Design review of the part built by this model. Coordinates are the model's own, in mm. Face numbers are marked on the shaded views. Coordinates: 2 decimals unless noted, no trailing zeros. Order: outer loops, then holes, each group sorted by start corner. A loop starts at its lowest first (then second) coordinate and runs counter-clockwise, first axis right, second up. Notation, with made-up numbers: (16, 12) -> (52, 12) arc R12 ccw to (52, 18) -> close; hole circle Ø5 at (86.25, 1.25). An arc over 180 degrees is marked (long way). Write item = value, one per line.
```python
from build123d import *

# Parameters (mm, degrees)
SKETCH_1_W          = 48.12
SKETCH_1_H          = 12
SKETCH_1_R          = 0.85
SKETCH_1_W_2        = 5
EXTRUDE_1_DEPTH     = 1.6
CUT_EXTRUDE_1_DEPTH = 1.6
FILLET_1_R          = 1


with BuildPart() as part:
    # 草图1 → 凸台-拉伸1 (new body)
    # profile 1 of 2: a face of its own
    with BuildSketch(Plane.XY):
        with Locations((29.06, -6)):
            Rectangle(SKETCH_1_W, SKETCH_1_H)
        with Locations((50.62, -9)):
            Circle(SKETCH_1_R, mode=Mode.SUBTRACT)
        with Locations((50.62, -3)):
            Circle(SKETCH_1_R, mode=Mode.SUBTRACT)
    # profile 2 of 2: a face of its own
    with BuildSketch(Plane.XY):
        with Locations((2.5, -6)):
            Rectangle(SKETCH_1_W_2, SKETCH_1_H)
        with Locations((2.5, -9)):
            Circle(SKETCH_1_R, mode=Mode.SUBTRACT)
        with Locations((2.5, -3)):
            Circle(SKETCH_1_R, mode=Mode.SUBTRACT)
    extrude(amount=EXTRUDE_1_DEPTH)

    # 草图2 → 切除-拉伸1 (cut)
    with BuildSketch(Plane(origin=(0, 0, 0), x_dir=(-1, 0, 0), z_dir=(0, 0, -1))):
        with BuildLine():
            Line((-42.930819808, -3), (-10.189180192, -3))
            ThreePointArc((-10.189180192, -3), (-7.189180192, -6), (-10.189180192, -9))
            Line((-10.189180192, -9), (-42.930819808, -9))
            ThreePointArc((-42.930819808, -9), (-45.930819808, -6), (-42.930819808, -3))
        make_face()
    extrude(amount=-CUT_EXTRUDE_1_DEPTH, mode=Mode.SUBTRACT)

    # 圆角1
    fillet_1_edges = [part.edges().sort_by_distance(p)[0] for p in [
        (53.12, -12, 0.8),
        (0, -12, 0.8),
        (0, 0, 0.8),
        (53.12, 0, 0.8),
    ]]
    fillet(fillet_1_edges, radius=FILLET_1_R)


solid = part.part
```
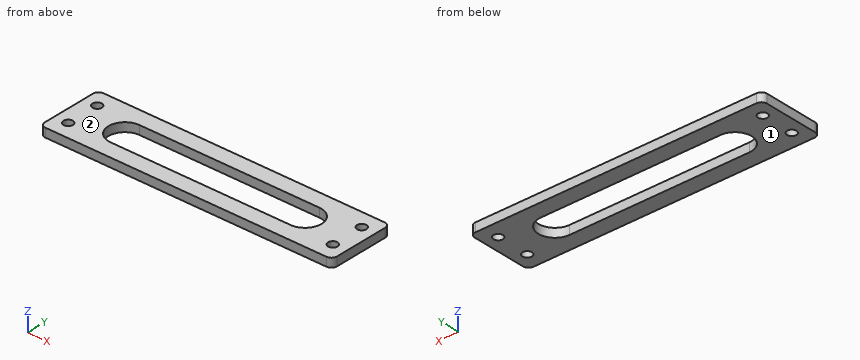
(1) We need section D-D (x = 50.62). Write out the cut boundary in (y, z), and give its area (3 significant figures).
Report:
outline = (-12, 0) -> (-9.85, 0) -> (-9.85, 1.6) -> (-12, 1.6) -> close; (-8.15, 0) -> (-3.85, 0) -> (-3.85, 1.6) -> (-8.15, 1.6) -> close; (-2.15, 0) -> (0, 0) -> (0, 1.6) -> (-2.15, 1.6) -> close
area = 13.8 mm²
(2) We need section A-A (x = 40.5). Write out the cut boundary in (y, z).
Report:
outline = (-12, 0) -> (-9, 0) -> (-9, 1.6) -> (-12, 1.6) -> close; (-3, 0) -> (0, 0) -> (0, 1.6) -> (-3, 1.6) -> close
(3) We need section B-B (y = -6). Write out the cut boundary in (x, z), and give its area (3 significant figures).
Report:
outline = (0, 0) -> (7.19, 0) -> (7.19, 1.6) -> (0, 1.6) -> close; (45.93, 0) -> (53.12, 0) -> (53.12, 1.6) -> (45.93, 1.6) -> close
area = 23.0 mm²
(4) The part is to be moulded in two halves that separate along Z. For the marked faces 1 and 2, say which applies: released by +Z, released by -Z, zero draft, split by the parting line, or undercut.
Report:
face_1 = released by -Z
face_2 = released by +Z
(5) For L1, parallel to Y at x = 2.5, z = 1.1; L2, parallel to Y at x = 28, z = 0.1; L3, parallel to X at y = -2.5, z = 0.75, list the stretches that pass through material, from the lowest coordinate up.
Report:
L1 = -12 to -9.85, -8.15 to -3.85, -2.15 to 0
L2 = -12 to -9, -3 to 0
L3 = 0 to 1.81, 3.19 to 49.93, 51.31 to 53.12
(6) We need section C-C (z = 0.3). Write out the cut boundary in (x, y).
Report:
outline = (0, -11) arc R1 ccw to (1, -12) -> (52.12, -12) arc R1 ccw to (53.12, -11) -> (53.12, -1) arc R1 ccw to (52.12, 0) -> (1, 0) arc R1 ccw to (0, -1) -> close; hole circle Ø1.7 at (2.5, -9); hole circle Ø1.7 at (2.5, -3); hole (10.19, -9) -> (42.93, -9) arc R3 ccw to (42.93, -3) -> (10.19, -3) arc R3 ccw to start; hole circle Ø1.7 at (50.62, -9); hole circle Ø1.7 at (50.62, -3)
